```python
from build123d import *

# Parameters (mm, degrees)
RESSALTO_EXTRUS_O1_DEPTH      = 3.5
RESSALTO_EXTRUS_O2_DEPTH      = 1
RESSALTO_EXTRUS_O3_DEPTH      = 10
RESSALTO_EXTRUS_O3_DEPTH_BACK = 10
ESBO_O4_W                     = 26.5
ESBO_O4_H                     = 8
CORTE_EXTRUS_O1_DEPTH         = 7
CORTE_EXTRUS_O2_START         = -20
ESBO_O4_2_W                   = 26.5
ESBO_O4_2_H                   = 8
CORTE_EXTRUS_O2_DEPTH         = 7
CORTE_EXTRUS_O3_DEPTH         = 71.418925013
CORTE_EXTRUS_O3_DEPTH_BACK    = 71.418925013
ESBO_O5_R                     = 1.5
FILETE1_R                     = 2
FILETE2_R                     = 2.5
FILETE3_R                     = 1.5
CORTE_EXTRUS_O4_DEPTH         = 7
CORTE_EXTRUS_O5_START         = -13
CORTE_EXTRUS_O5_DEPTH         = 7


with BuildPart() as part:
    # Esboço1 → Ressalto-extrusão1 (new body)
    with BuildSketch(Plane(origin=(0, 0, 0), x_dir=(1, 0, 0), z_dir=(0, 1, 0))):
        Polygon((-16.05, 20.15), (16.05, 20.15), (16.05, 15.05), (43.05, 15.05), (43.05, -15.05), (-43.05, -15.05), (-43.05, 15.05), (-16.05, 15.05), align=None)
        Polygon((12.05, 11.05), (39.05, 11.05), (39.05, -11.05), (-39.05, -11.05), (-39.05, 11.05), (-12.05, 11.05), (-12.05, 16.15), (12.05, 16.15), align=None, mode=Mode.SUBTRACT)
    extrude(amount=RESSALTO_EXTRUS_O1_DEPTH)

    # Esboço2 → Ressalto-extrusão2 (add)
    with BuildSketch(Plane.XZ):
        Polygon((39.05, 11.05), (39.05, -11.05), (12.05, -11.05), (12.05, -16.15), (-12.05, -16.15), (-12.05, -11.05), (-39.05, -11.05), (-39.05, 11.05), align=None)
        Polygon((38.05, -10.05), (38.05, 10.05), (-38.05, 10.05), (-38.05, -10.05), (-11.05, -10.05), (-11.05, -15.15), (11.05, -15.15), (11.05, -10.05), align=None, mode=Mode.SUBTRACT)
    extrude(amount=-RESSALTO_EXTRUS_O2_DEPTH)

    # Esboço3 → Ressalto-extrusão3 (add, two sides: drawn at the far end of the back side and taken through both)
    with BuildSketch(Plane(origin=(0, 0, 0), x_dir=(0, 0, -1), z_dir=(1, 0, 0)).offset(-RESSALTO_EXTRUS_O3_DEPTH_BACK)):
        Polygon((20.15, 0), (28.65, 0), (55.15, 8), (55.15, 11.5), (25.15, 11.5), (25.15, 3.5), (20.15, 3.5), align=None)
        Polygon((28.65, 3.5), (43.55625, 8), (28.65, 8), align=None, mode=Mode.SUBTRACT)
    extrude(amount=RESSALTO_EXTRUS_O3_DEPTH + RESSALTO_EXTRUS_O3_DEPTH_BACK)

    # Esboço4 → Corte-extrusão1 (cut)
    with BuildSketch(Plane(origin=(10, 0, 0), x_dir=(0, 0, -1), z_dir=(1, 0, 0))):
        with Locations((41.9, 4)):
            Rectangle(ESBO_O4_W, ESBO_O4_H)
    extrude(amount=-CORTE_EXTRUS_O1_DEPTH, mode=Mode.SUBTRACT)

    # Esboço4<2> → Corte-extrusão2 (cut)
    with BuildSketch(Plane(origin=(10, 0, 0), x_dir=(0, 0, -1), z_dir=(1, 0, 0)).offset(CORTE_EXTRUS_O2_START)):
        with Locations((41.9, 4)):
            Rectangle(ESBO_O4_2_W, ESBO_O4_2_H)
    extrude(amount=CORTE_EXTRUS_O2_DEPTH, mode=Mode.SUBTRACT)

    # Esboço5 → Corte-extrusão3 (cut, two sides: drawn at the far end of the back side and taken through both)
    with BuildSketch(Plane.XZ.offset(-8).offset(-CORTE_EXTRUS_O3_DEPTH_BACK)):
        with Locations(Location((-6.5, -45.15, 0), (0, 0, 270))):
            Circle(ESBO_O5_R)
        with Locations(Location((6.5, -45.15, 0), (0, 0, 270))):
            Circle(ESBO_O5_R)
        with Locations(Location((-6.5, -35.15, 0), (0, 0, 270))):
            Circle(ESBO_O5_R)
        with Locations(Location((6.5, -35.15, 0), (0, 0, 270))):
            Circle(ESBO_O5_R)
    extrude(amount=CORTE_EXTRUS_O3_DEPTH + CORTE_EXTRUS_O3_DEPTH_BACK, mode=Mode.SUBTRACT)

    # Filete1
    filete1_edges = [part.edges().sort_by_distance(p)[0] for p in [
        (39.05, 2.25, 11.05),
        (39.05, 2.25, -11.05),
        (12.05, 2.25, -11.05),
        (12.05, 2.25, -16.15),
        (-12.05, 2.25, -16.15),
        (-12.05, 2.25, -11.05),
        (-39.05, 2.25, -11.05),
        (-39.05, 2.25, 11.05),
    ]]
    fillet(filete1_edges, radius=FILETE1_R)

    # Filete2
    filete2_edges = [part.edges().sort_by_distance(p)[0] for p in [
        (10, 1.75, -20.15),
        (-10, 1.75, -20.15),
        (-16.05, 1.75, -20.15),
        (16.05, 1.75, -20.15),
        (16.05, 1.75, -15.05),
        (43.05, 1.75, -15.05),
        (43.05, 1.75, 15.05),
        (-43.05, 1.75, 15.05),
        (-43.05, 1.75, -15.05),
        (-16.05, 1.75, -15.05),
    ]]
    fillet(filete2_edges, radius=FILETE2_R)

    # Filete3
    filete3_edges = [part.edges().sort_by_distance(p)[0] for p in [
        (10, 9.75, -55.15),
        (-10, 9.75, -55.15),
        (0, 11.5, -25.15),
        (0, 3.5, -25.15),
        (0, 8, -28.65),
        (0, 8, -43.55625),
        (0, 3.5, -28.65),
    ]]
    fillet(filete3_edges, radius=FILETE3_R)

    # Esboço6 → Corte-extrusão4 (cut)
    with BuildSketch(Plane(origin=(10, 0, 0), x_dir=(0, 0, -1), z_dir=(1, 0, 0))):
        with BuildLine():
            Line((26.15, 0), (28.65, 0))
            Line((28.65, 0), (28.65, 2.5))
            ThreePointArc((28.65, 2.5), (27.917766953, 0.732233047), (26.15, 0))
        make_face()
    extrude(amount=-CORTE_EXTRUS_O4_DEPTH, mode=Mode.SUBTRACT)

    # Esboço6<2> → Corte-extrusão5 (cut)
    with BuildSketch(Plane(origin=(10, 0, 0), x_dir=(0, 0, -1), z_dir=(1, 0, 0)).offset(CORTE_EXTRUS_O5_START)):
        with BuildLine():
            Line((26.15, 0), (28.65, 0))
            Line((28.65, 0), (28.65, 2.5))
            ThreePointArc((28.65, 2.5), (27.917766953, 0.732233047), (26.15, 0))
        make_face()
    extrude(amount=-CORTE_EXTRUS_O5_DEPTH, mode=Mode.SUBTRACT)


solid = part.part
```
The listing builds one solid part. Answer for the finished solid, in the listing's coordinates (mm). A direction names the side the tool comes from. Round coordinates to 2 decimals unless told otherwise and drop trailing zeros. Order: outer loops, then holes, each group sorted by start corner. A loop starts at its lowest first (then second) coordinate and runs counter-clockwise, first axis right, second up. Notation, with made-up numbers: (-18.5, 87.25) - (-1.5, 87.25) arc R35 cw to (-1.5, 123.25) - close; hole circle Ø11 at (-20, -4.5). An arc over 180 degrees is marked (long way). Put each result on its own line as item: value. Start each with the question number.
(1) For faces 1 (the flat face through (0, 8, -25.15)), 2 (the flat face through (-26, 2, -11.05)), 3 (the flat face through (10, 8.4, -34.5)), 4 (the cylindrical face through (6.549, 0.752, -27.937)), 5 (the cylindrical face through (-6.451, 0.752, -27.937)), determine the directions among +Z, -Z, +X, -X, +Y, -Y from which every point of the face is accessible in a straight line to the end or side of a thin tool.
(2) Find section A-A (x = -29.5). Give the vertices of the cut face in (y, z), plus the area to 3 significant figures.
(3) Straight lines are drawn through the part: probe 1 along Z at (x, y) = (-6.5, 9.6); probe 2 along X at (y, z) = (10.5, -45.15); probe 3 along Z at (x, y) = (-34.5, 3). For each, find the intervals that lie inside material, in ascending order. Write a range as from..to.
(4) Find section D-D (z = -48). Give the vertices of the cut face in (x, y), plus the area to 3 significant figures.
(5) Given P1, Ø0.8, axis at x = -12.5, y = 0.5, coming from the -Z side; P2, Ø1.8, axis at x = 26.5, y = 2.5, coming from the -Z side; P3, Ø22, axis at x = 3, z = -46.5, coming from the -Y side, each flat-ended and moving along its own axis, determine where each tip first touches the part or whether it passes through.
(6) Find section B-B (z = 5.5). Give the vertices of the cut face in (x, y).
(7) Determine the mould class of faces 6 (the cylindrical face through (-7.075, 9.775, -36.536)), 7 (the cylindrical face through (16.763, 1.774, -15.802)), 8 (the flat face through (-43.05, 2, 0)), 9 (the flat face through (0, 2, -16.15)) for opening direction Z: released by +Z, released by -Z, zero draft, split by the parting line, or undercut.
(8) Find section C-C (x = 6.5). Give the vertices of the cut face in (y, z).
Reply:
1. face 1: +Z, +X, -X, +Y
1. face 2: +Y
1. face 3: -Z, +X, +Y, -Y
1. face 4: -Z, +X, -Y
1. face 5: -Z, -X, -Y
2. outline: (0, -15.05) - (3.5, -15.05) - (3.5, -11.05) - (1, -11.05) - (1, -10.05) - (0, -10.05) - close; (0, 10.05) - (1, 10.05) - (1, 11.05) - (3.5, 11.05) - (3.5, 15.05) - (0, 15.05) - close
2. area: 30.0 mm^2
3. probe 1: -55.15..-46.65, -43.65..-36.65, -33.65..-25.15
3. probe 2: -10..-8, -5..5, 8..10
3. probe 3: -15.05..-11.05, 11.05..15.05
4. outline: (-10, 8) - (-3, 8) - (-3, 5.84) - (3, 5.84) - (3, 8) - (10, 8) - (10, 11.5) - (-10, 11.5) - close
4. area: 83.0 mm^2
5. P1: z = -20.18
5. P2: z = -15.05
5. P3: y = 2.07
6. outline: (-43.05, 0) - (-38.05, 0) - (-38.05, 1) - (-39.05, 1) - (-39.05, 3.5) - (-43.05, 3.5) - close; (38.05, 0) - (43.05, 0) - (43.05, 3.5) - (39.05, 3.5) - (39.05, 1) - (38.05, 1) - close
7. face 6: undercut
7. face 7: released by -Z
7. face 8: zero draft
7. face 9: undercut
8. outline: (0, -26.15) arc R2.5 ccw to (2.5, -28.65) - (6.5, -28.65) arc R1.5 cw to (8, -30.15) - (8, -33.65) - (11.5, -33.65) - (11.5, -26.65) arc R1.5 ccw to (10, -25.15) - (5, -25.15) arc R1.5 cw to (3.5, -23.65) - (3.5, -16.15) - (1, -16.15) - (1, -15.15) - (0, -15.15) - close; (0, 10.05) - (1, 10.05) - (1, 11.05) - (3.5, 11.05) - (3.5, 15.05) - (0, 15.05) - close; (8, -55.15) - (11.5, -55.15) - (11.5, -46.65) - (8, -46.65) - close; (8, -43.65) - (11.5, -43.65) - (11.5, -36.65) - (8, -36.65) - close
